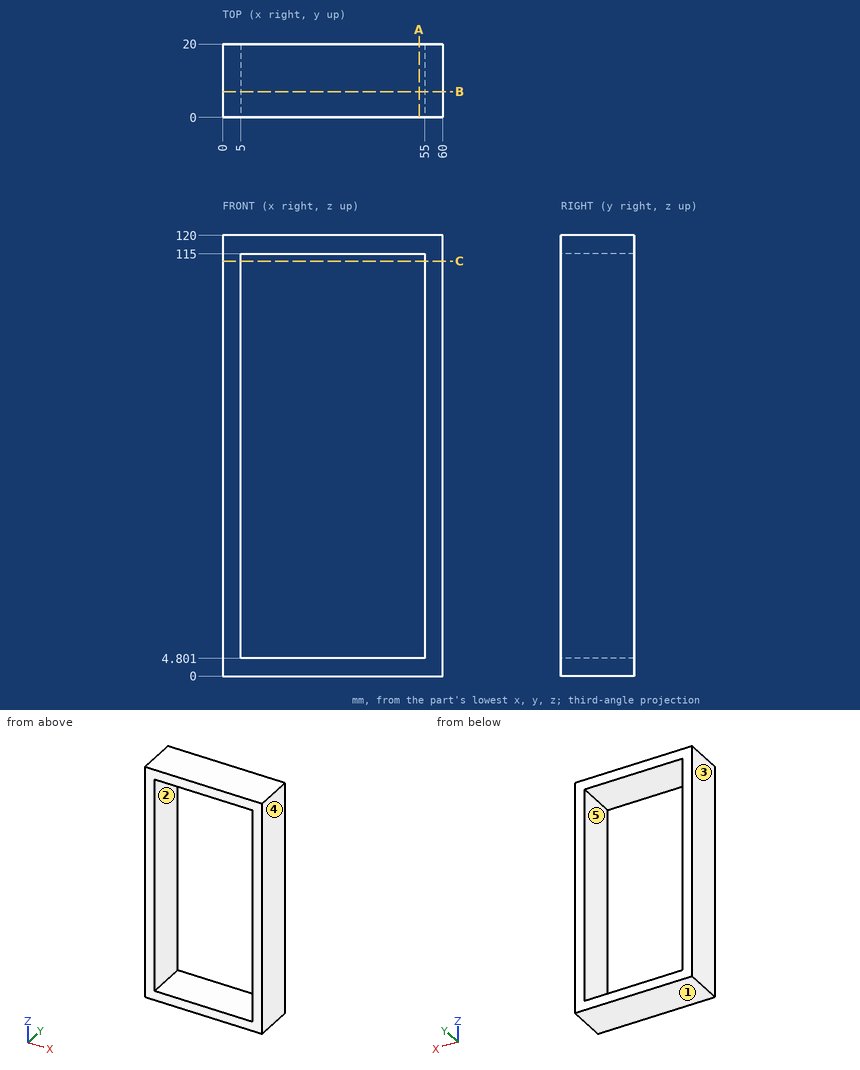
Geometry check sheet. Reference: drawing and pictorial views, mm from the part's lowest x, y, z. A direction names the side the tool comes from. Give positions to 0.01 mm unless a question says otherwise; leave off trailing zeros. Loops run counter-clockwise (first coordinate to the right, second up) from the corner with the lowest first, then second, coordinate; pieces in that order, holes last. Notation, with made-up numbers: (-3.75, 29) - (0.25, 29) arc R25 ccw to (0.25, 44) - close; hole circle Ø4 at (63.5, -15.5). An arc over 180 degrees is marked (long way). Use CSV: the item, a comma, the result in double quotes. Start each with the question number.
Q1. Scan lines: probe 1 along Z at (x, y) = (16, 13.5); probe 2 along X at (y, z) = (12, 71.5). Record each from-to range of solid material in increasing order. Write a range as from..to.
Q2. Release check for a two-part mould opening along Z. For the marked faces 1, 2 and 3 record: +Z half, -Z half, draft (parallel to the pull), parting line (faces both ways), or undercut.
Q3. Section check A-A, the plane x = 53.5. Record the cut outline in (y, z), and give its area (3 significant figures).
Q4. Section check C-C, the plane z = 113. Record the cut outline in (x, y), and give its area (3 significant figures).
Q5. Access from +Z, -Z, +X, -X, +Y, -Y to the whole of each face (thin tool, end or side, straight path). Record for the marked faces 4 and 5.
Q6. Section check B-B, the plane y = 7. Record the cut outline in (x, z).
Findings below:
1,probe 1,"z = 0..4.8, 115..120"
1,probe 2,"x = 0..5, 55..60"
2,face 1,"-Z half"
2,face 2,"undercut"
2,face 3,"draft"
3,outline,"(0, 0) - (20, 0) - (20, 4.8) - (0, 4.8) - close; (0, 115) - (20, 115) - (20, 120) - (0, 120) - close"
3,area,"196 mm^2"
4,outline,"(0, 0) - (5, 0) - (5, 20) - (0, 20) - close; (55, 0) - (60, 0) - (60, 20) - (55, 20) - close"
4,area,"200 mm^2"
5,face 4,"+Z, -Z, +X, +Y, -Y"
5,face 5,"+Y, -Y"
6,outline,"(0, 0) - (60, 0) - (60, 120) - (0, 120) - close; hole (5, 4.8) - (55, 4.8) - (55, 115) - (5, 115) - close"
